For this review, take the finished solid that the model builds, in its own axes (mm). A direction names the side the tool comes from. Coordinates: 2 decimals unless noted, no trailing zeros. Order: outer loops, then holes, each group sorted by start corner. A loop starts at its lowest first (then second) coordinate and runs counter-clockwise, first axis right, second up. Notation, with made-up numbers: (-23, 7.5) -> (-8, 7.5) arc R19 cw to (-8, 20.5) -> close; hole circle Ø9 at (54.25, 37.5). An arc over 180 degrees is marked (long way). Answer as a JSON object with one key per item and string values. Group by question number.
1) Wall thickness on L1, parallel to X at y = -0.3, z = 3.25; L2, parallel to Z at x = 7.25, y = 0.75; L3, parallel to Z at x = 13.75, y = -0.3: over which ranges is each line inside the solid? List them lowest first.
2) Add section A-A, the plane z = -3. Write out the cut boundary in (x, y).
3) Add section B-B, the plane y = -0.6. Write out the cut boundary in (x, z).
4) For pin 1 (1 mm diameter, centred on y = -0.5, z = -2, fed in from -X); pin 2 (1 mm diameter, centred on x = 6, y = 0, fed in from -Z), all flat-tipped, find the tip position at first contact; note any pin that passes through.
5) Add section D-D, the plane x = 13. Write out the cut boundary in (y, z).
6) Add section C-C, the plane x = 9.25. Write out the cut boundary in (y, z).
7) Machinability: for faces 1 (the flat face through (16, 0, 0)), 2 (the flat face through (4, 0, 4)), 3 (the flat face through (8, 0, -2)), which of the approach directions +Z, -Z, +X, -X, +Y, -Y give a long, thin tool a straight path to every point of the face, cutting with its end or side? Answer none if there is none.
8) Draft analysis for pull direction X (two halves, no side actions). For faces 4 (the cylindrical face through (2, 0, -5)), 5 (the flat face through (0, 0, 0)), 6 (the flat face through (4, 0, -3)), state which applies: +X half, -X half, draft (parallel to the pull), parting line (faces both ways), or undercut.
from build123d import *

# Parameters (mm, degrees)
EXTRUDE_1_DEPTH     = 16
SKETCH_2_W          = 8
SKETCH_2_H          = 9.708819165
SKETCH_2_H_2        = 9.650339741
CUT_EXTRUDE_1_DEPTH = 14


with BuildPart() as part:
    # 草图1 → 凸台-拉伸1 (new body)
    with BuildSketch(Plane(origin=(0, 0, 0), x_dir=(0, 0, -1), z_dir=(1, 0, 0))):
        with BuildLine():
            Line((-4, 1), (4, 1))
            ThreePointArc((4, 1), (5, 0), (4, -1))
            Line((4, -1), (-4, -1))
            ThreePointArc((-4, -1), (-5, 0), (-4, 1))
        make_face()
    extrude(amount=EXTRUDE_1_DEPTH)

    # 草图2 → 切除-拉伸1 (cut)
    with BuildSketch(Plane(origin=(0, 1, 0), x_dir=(1, 0, 0), z_dir=(0, 1, 0))):
        with Locations((8, 6.854409583)):
            Rectangle(SKETCH_2_W, SKETCH_2_H)
        with Locations((8, -6.825169871)):
            Rectangle(SKETCH_2_W, SKETCH_2_H_2)
    extrude(amount=-CUT_EXTRUDE_1_DEPTH, mode=Mode.SUBTRACT)


solid = part.part
Output values:
{
 "1": {"L1": "x = 0 to 4, 12 to 16", "L2": "z = -2 to 2", "L3": "z = -4.95 to 4.95"},
 "2": {"outline": "(0, -1) -> (4, -1) -> (4, 1) -> (0, 1) -> close; (12, -1) -> (16, -1) -> (16, 1) -> (12, 1) -> close"},
 "3": {"outline": "(0, -4.8) -> (4, -4.8) -> (4, -2) -> (12, -2) -> (12, -4.8) -> (16, -4.8) -> (16, 4.8) -> (12, 4.8) -> (12, 2) -> (4, 2) -> (4, 4.8) -> (0, 4.8) -> close"},
 "4": {"pin 1": "stops at x = 0", "pin 2": "stops at z = -2"},
 "5": {"outline": "(-1, -4) arc R1 ccw to (1, -4) -> (1, 4) arc R1 ccw to (-1, 4) -> close"},
 "6": {"outline": "(-1, -2) -> (1, -2) -> (1, 2) -> (-1, 2) -> close"},
 "7": {"face 1": "+Z, -Z, +X, +Y, -Y", "face 2": "+Z, +Y, -Y", "face 3": "-Z, +Y, -Y"},
 "8": {"face 4": "draft", "face 5": "-X half", "face 6": "undercut"}
}
